Build history of the part. All positions in model axes, mm. Round coordinates to 2 decimals unless told otherwise and drop trailing zeros. Order: outer loops, then holes, each group sorted by start corner. A loop starts at its lowest first (then second) coordinate and runs counter-clockwise, first axis right, second up. Notation, with made-up numbers: (5, 7) -> (31, 7) arc R18 ccw to (31, 39) -> close; hole circle Ø11 at (8, 15.25). An arc over 180 degrees is marked (long way). Answer as a JSON object with one key per item and string values.
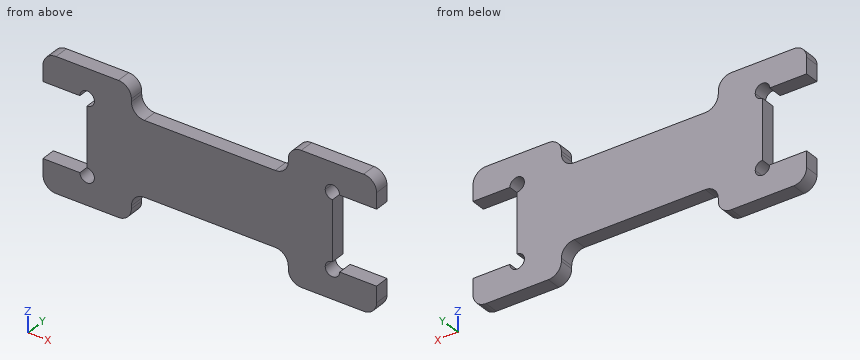
from build123d import *

# Parameters (mm, degrees)
BOSS_EXTRUDE1_DEPTH = 5
FILLET1_R           = 4.5


with BuildPart() as part:
    # Sketch1 → Boss-Extrude1 (new body)
    with BuildSketch(Plane(origin=(0, 0, 0), x_dir=(1, 0, 0), z_dir=(0, 1, 0))):
        with BuildLine():
            ThreePointArc((-44.85, 12.8), (-42.35, 15.3), (-39.85, 12.8))
            Line((-39.85, 12.8), (-27.09, 12.8))
            Line((-27.09, 12.8), (-27.09, 22.8))
            Line((-27.09, 22.8), (-57.61, 22.8))
            Line((-57.61, 22.8), (-57.61, 12.8))
            Line((-57.61, 12.8), (-44.85, 12.8))
        make_face()
        with BuildLine():
            ThreePointArc((-42.35, -10.3), (-40.582233047, -11.032233047), (-39.85, -12.8))
            Line((-39.85, -12.8), (-27.09, -12.8))
            Line((-27.09, -12.8), (27.09, -12.8))
            Line((27.09, -12.8), (39.85, -12.8))
            ThreePointArc((39.85, -12.8), (40.582233047, -11.032233047), (42.35, -10.3))
            Line((42.35, -10.3), (42.35, 10.3))
            ThreePointArc((42.35, 10.3), (40.582233047, 11.032233047), (39.85, 12.8))
            Line((39.85, 12.8), (27.09, 12.8))
            Line((27.09, 12.8), (-27.09, 12.8))
            Line((-27.09, 12.8), (-39.85, 12.8))
            ThreePointArc((-39.85, 12.8), (-40.582233047, 11.032233047), (-42.35, 10.3))
            Line((-42.35, 10.3), (-42.35, -10.3))
        make_face()
        with BuildLine():
            Line((-44.85, -12.8), (-57.61, -12.8))
            Line((-57.61, -12.8), (-57.61, -22.8))
            Line((-57.61, -22.8), (-27.09, -22.8))
            Line((-27.09, -22.8), (-27.09, -12.8))
            Line((-27.09, -12.8), (-39.85, -12.8))
            ThreePointArc((-39.85, -12.8), (-42.35, -15.3), (-44.85, -12.8))
        make_face()
        with BuildLine():
            Line((39.85, -12.8), (27.09, -12.8))
            Line((27.09, -12.8), (27.09, -22.8))
            Line((27.09, -22.8), (57.61, -22.8))
            Line((57.61, -22.8), (57.61, -12.8))
            Line((57.61, -12.8), (44.85, -12.8))
            ThreePointArc((44.85, -12.8), (42.35, -15.3), (39.85, -12.8))
        make_face()
        with BuildLine():
            Line((27.09, 22.8), (27.09, 12.8))
            Line((27.09, 12.8), (39.85, 12.8))
            ThreePointArc((39.85, 12.8), (42.35, 15.3), (44.85, 12.8))
            Line((44.85, 12.8), (57.61, 12.8))
            Line((57.61, 12.8), (57.61, 22.8))
            Line((57.61, 22.8), (27.09, 22.8))
        make_face()
    extrude(amount=BOSS_EXTRUDE1_DEPTH)

    # Fillet1
    fillet1_edges = [part.edges().sort_by_distance(p)[0] for p in [
        (-57.61, 2.5, -22.8),
        (-27.09, 2.5, -22.8),
        (-27.09, 2.5, -12.8),
        (27.09, 2.5, -12.8),
        (27.09, 2.5, -22.8),
        (57.61, 2.5, -22.8),
        (57.61, 2.5, 22.8),
        (27.09, 2.5, 22.8),
        (27.09, 2.5, 12.8),
        (-27.09, 2.5, 12.8),
        (-27.09, 2.5, 22.8),
        (-57.61, 2.5, 22.8),
    ]]
    fillet(fillet1_edges, radius=FILLET1_R)


solid = part.part
1) Cut at A-A, the plane x = 50. Give the cut face in (y, z), plus the area to 3 significant figures.
Checked values:
{"outline": "(0, -22.8) -> (5, -22.8) -> (5, -12.8) -> (0, -12.8) -> close; (0, 12.8) -> (5, 12.8) -> (5, 22.8) -> (0, 22.8) -> close", "area": "100 mm²"}
2) Cut at C-C, the plane x = -19.5. Give the cut face in (y, z), plus the area to 3 significant figures.
Checked values:
{"outline": "(0, -12.8) -> (5, -12.8) -> (5, 12.8) -> (0, 12.8) -> close", "area": "128 mm²"}
3) Flat gauge pins, fed straight in: pin 1 Ø3 at (y, z) = (3, -7.5) entering from -X; pin 2 Ø2.5 at (y, z) = (2.5, 2.5) entering from +X; pin 3 Ø1.5 at (x, y) = (53.5, 2) entering from +Z; pin 4 Ø1.5 at (x, y) = (-9, 1.5) entering from -Z. Where does each tip first touch, or does it go through?
Checked values:
{"pin 1": "stops at x = -42.35", "pin 2": "stops at x = 42.35", "pin 3": "stops at z = 22.8", "pin 4": "stops at z = -12.8"}
4) Probe L1, parallel to X at y = 2.6, z = -17.5; L2, parallel to Z at x = 49, y = 0.6; L3, parallel to X at y = 0.95, z = -0.5. List the from-to ranges inside material, lowest first. Write a range as from..to.
Checked values:
{"L1": "x = -57.61..-27.09, 27.09..57.61", "L2": "z = -22.8..-12.8, 12.8..22.8", "L3": "x = -42.35..42.35"}
5) Cut at B-B, the plane z = -3. Give the cut face in (x, y).
Checked values:
{"outline": "(-42.35, 0) -> (42.35, 0) -> (42.35, 5) -> (-42.35, 5) -> close"}
